The listing builds one solid part. Answer for the finished solid, in the listing's coordinates (mm). A direction names the side the tool comes from. Give positions to 0.01 mm unless a question says otherwise; leave off trailing zeros. Write each loop counter-clockwise with the first axis right and the second up, starting at its lowest first coordinate (ties: lowest second). Pieces come first, ordered by that corner, then holes. Notation, with made-up numbers: (1.25, -18.75) - (5.25, -18.75) arc R16 ccw to (5.25, 5.25) - close; hole circle Ø3 at (62, -34.75). An arc over 180 degrees is marked (long way). Answer in a Markdown table with one row per item. Add a question column.
Autodesk Inventor part; units mm, degrees
ref_plane "Start Plane" through (0, 0, 80) normal (0, 0, 1) x (1, 0, 0)
ref_plane "End Plane" through (0, 0, 435) normal (0, 0, 1) x (1, 0, 0)
ref_plane "YZ Plane" through (0, 0, 0) normal (1, 0, 0) x (0, 1, 0)
ref_plane "Start Plane" through (0, 0, 80) normal (0, 0, 1) x (1, 0, 0)
ref_plane "End Plane" through (0, 0, 435) normal (0, 0, 1) x (1, 0, 0)
sketch "Sketch" plane through (0, 0, 0) normal (0, 0, 1) x (1, 0, 0)
  line L0 (-20, -34) -> (-20, 34)
  line L1 (-14, 40) -> (14, 40)
  line L2 (20, 34) -> (20, -34)
  line L3 (14, -40) -> (-14, -40)
  arc A0 (-20, -34) -> (-14, -40) centre (-14, -34) ccw
  arc A1 (20, 34) -> (14, 40) centre (14, 34) ccw
  arc A2 (-14, 40) -> (-20, 34) centre (-14, 34) ccw
  arc A3 (14, -40) -> (20, -34) centre (14, -34) ccw
  arc A4 (-14, 37) -> (-17, 34) centre (-14, 34) ccw
  line L4 (-14, 37) -> (14, 37)
  arc A5 (17, 34) -> (14, 37) centre (14, 34) ccw
  line L5 (17, 34) -> (17, -34)
  arc A6 (14, -37) -> (17, -34) centre (14, -34) ccw
  line L6 (14, -37) -> (-14, -37)
  arc A7 (-17, -34) -> (-14, -37) centre (-14, -34) ccw
  line L7 (-17, -34) -> (-17, 34)
  line L8 (0, 57.7397) -> (0, -57.7397) construction
  line L9 (-29.7397, 0) -> (29.7397, 0) construction
  dimension "d7" = 6
  dimension "d9" = 40
  dimension "d11" = 80
  dimension "d12" = 3
  dimension "d15" = 20
  dimension "d16" = 40
extrude "Body" add sketch "Sketch" along normal up to surface (355 mm away) from surface at 80
sketch "Sketch3" plane through (0, 0, 0) normal (0, 0, 1) x (1, 0, 0)
  line L0 (0, 0) -> (10, 0)
ref_plane "Work Plane3" through (0, 0, 0) normal (0, -1, 0) x (1, 0, 0)
sketch "Sketch4" plane through (0, 0, 0) normal (0, -1, 0) x (1, 0, 0)
  line L0 (-2, 80) -> (12, 80)
  line L1 (-2, 435) -> (12, 435)
  dimension "d18" = 355
equation "\"d7\" = G_IR"
equation "\"d9\" = G_W"
equation "\"d11\" = G_H"
equation "\"d12\" = G_T"
equation "\"d15\" = 0.5 * d9"
equation "\"d16\" = 0.5 * d11"
equation "\"d3\" = G_L"
equation "\"G_W\" = 40"
equation "\"G_H\" = 80"
equation "\"G_T\" = 3"
equation "\"G_IR\" = 6"
equation "\"G_L\" = d18"
equation "\"d14\" = G_OFFSET_END + B_L"
equation "\"B_L\" = 455"
properties part number "ISO 10799-2 - 80x40x3 - 355" material "Steel, Mild"
1. Section A-A (y = -11.5) is taken. Give the vertices of the cut face in (x, z).
2. The mould has two halves that part along Y. Classify faces 3 (the face through (0, -40, 255)), 4 (the face through (-18, 0, 80)), 5 (the face through (-17, 0, 255)): +Y half, -Y half, draft (parallel to the pull), parting line (faces both ways), or undercut.
3. A tool of negligible diameter and unlimited length cuts with its end or side. For faces 1 (the face through (0, 37, 255)), 2 (the face through (-18.196, -38.289, 255.015)), from which of +Z, -Z, +X, -X, +Y, -Y can it reach the whole face along a straight path? Write none if from no direction.
4. Section B-B (x = 7.5) is taken. Give the vertices of the cut face in (y, z).
5. Section C-C (z = 304) is taken. Give the vertices of the cut face in (x, y), and give its area (3 significant figures).
6. Given pin 1 Ø8 at (x, y) = (12, 21.5) entering from +Z; pin 2 Ø3 at (x, z) = (-16, 125.5) entering from -Y, each flat-ended and moving along its own axis, determine where each tip first touches the part or whether it passes through.
7. Straight lines are drawn through the part: L1, parallel to Y at x = -4, z = 354; L2, parallel to X at y = -28, z = 394. For each, find the intervals that lie inside material, in ascending order. Write a range as [from, to].
Geometry check:
| question | item | result |
|---|---|---|
| 1 | outline | (-20, 80) - (-17, 80) - (-17, 435) - (-20, 435) - close; (17, 80) - (20, 80) - (20, 435) - (17, 435) - close |
| 2 | face 3 | -Y half |
| 2 | face 4 | draft |
| 2 | face 5 | undercut |
| 3 | face 1 | +Z, -Z |
| 3 | face 2 | +Z, -Z, -X, -Y |
| 4 | outline | (-40, 80) - (-37, 80) - (-37, 435) - (-40, 435) - close; (37, 80) - (40, 80) - (40, 435) - (37, 435) - close |
| 5 | outline | (-20, -34) arc R6 ccw to (-14, -40) - (14, -40) arc R6 ccw to (20, -34) - (20, 34) arc R6 ccw to (14, 40) - (-14, 40) arc R6 ccw to (-20, 34) - close; hole (-17, -34) arc R3 ccw to (-14, -37) - (14, -37) arc R3 ccw to (17, -34) - (17, 34) arc R3 ccw to (14, 37) - (-14, 37) arc R3 ccw to (-17, 34) - close |
| 5 | area | 661 mm² |
| 6 | pin 1 | through |
| 6 | pin 2 | y = -39.98 |
| 7 | L1 | [-40, -37], [37, 40] |
| 7 | L2 | [-20, -17], [17, 20] |
